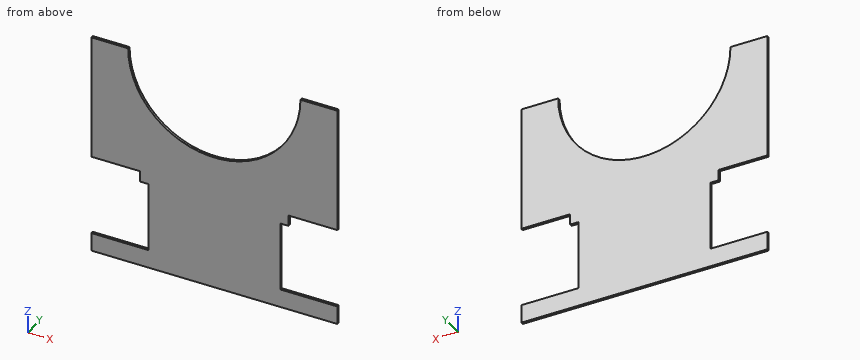
from build123d import *

# Parameters (mm, degrees)
EXTRUSION1_DEPTH = 3


with BuildPart() as part:
    # Esquisse1 → Extrusion1 (new body)
    with BuildSketch(Plane(origin=(0, 0, 0), x_dir=(1, 0, 0), z_dir=(0, 1, 0))):
        with BuildLine():
            Line((150, 0), (-150, 0))
            Line((-150, 0), (-150, -22))
            Line((-150, -22), (-80.5, -22))
            Line((-80.5, -22), (-80.5, -105))
            Line((-80.5, -105), (-90.5, -105))
            Line((-90.5, -105), (-90.5, -118))
            Line((-90.5, -118), (-150, -118))
            Line((-150, -118), (-150, -268))
            Line((-150, -268), (-105, -268))
            ThreePointArc((-105, -268), (0, -163), (105, -268))
            Line((105, -268), (150, -268))
            Line((150, -268), (150, -118))
            Line((150, -118), (90.5, -118))
            Line((90.5, -118), (90.5, -105))
            Line((90.5, -105), (80.5, -105))
            Line((80.5, -105), (80.5, -22))
            Line((80.5, -22), (150, -22))
            Line((150, -22), (150, 0))
        make_face()
    extrude(amount=EXTRUSION1_DEPTH)


solid = part.part
Build history of the part. All positions in model axes, mm. Round coordinates to 2 decimals unless told otherwise and drop trailing zeros. Write each loop counter-clockwise with the first axis right and the second up, starting at its lowest first coordinate (ties: lowest second). Pieces come first, ordered by that corner, then holes. Notation, with made-up numbers: M -7,-2 L 51,-2 A25 cw 51,35 Z; hole C -20.5,39 d9. An arc over 180 degrees is marked long. Answer as a JSON object with one key per item and string values. Group by question number.
(1) Cut at A-A (z = 241.5). Give the cut face in (x, y).
(2) Cut at B-B (x = 131). Give the cut face in (y, z).
(3) Drill centre lines: L1, parallel to X at y = 2.25, z = 100; L2, parallel to Z at x = 81, y = 1.9; L3, parallel to Z at x = 3, y = 1.35. Where is each one in solid material? Low to high.
(4) Flat gauge pins, fed straight in: pin 1 (0.9 mm diameter, centred on y = 2, z = 45, fed in from +X); pin 2 (1.5 mm diameter, centred on x = -73, y = 2.5, fed in from +Z). Where does each tip first touch, or does it go through?
(5) Cut at D-D (x = 0). Give the cut face in (y, z).
(6) Cut at C-C (y = 2.4). Give the cut face in (x, z), and give its area (3 significant figures).
Responses:
{
 "1": {"outline": "M -150,0 L -101.6,0 L -101.6,3 L -150,3 Z; M 101.6,0 L 150,0 L 150,3 L 101.6,3 Z"},
 "2": {"outline": "M 0,0 L 3,0 L 3,22 L 0,22 Z; M 0,118 L 3,118 L 3,268 L 0,268 Z"},
 "3": {"L1": "x = -80.5 to 80.5", "L2": "z = 0 to 22, 105 to 201.19", "L3": "z = 0 to 163.04"},
 "4": {"pin 1": "stops at x = 80.5", "pin 2": "stops at z = 193.26"},
 "5": {"outline": "M 0,0 L 3,0 L 3,163 L 0,163 Z"},
 "6": {"outline": "M -150,0 L 150,0 L 150,22 L 80.5,22 L 80.5,105 L 90.5,105 L 90.5,118 L 150,118 L 150,268 L 105,268 A105 cw -105,268 L -150,268 L -150,118 L -90.5,118 L -90.5,105 L -80.5,105 L -80.5,22 L -150,22 Z", "area": "50,000 mm2"}
}
